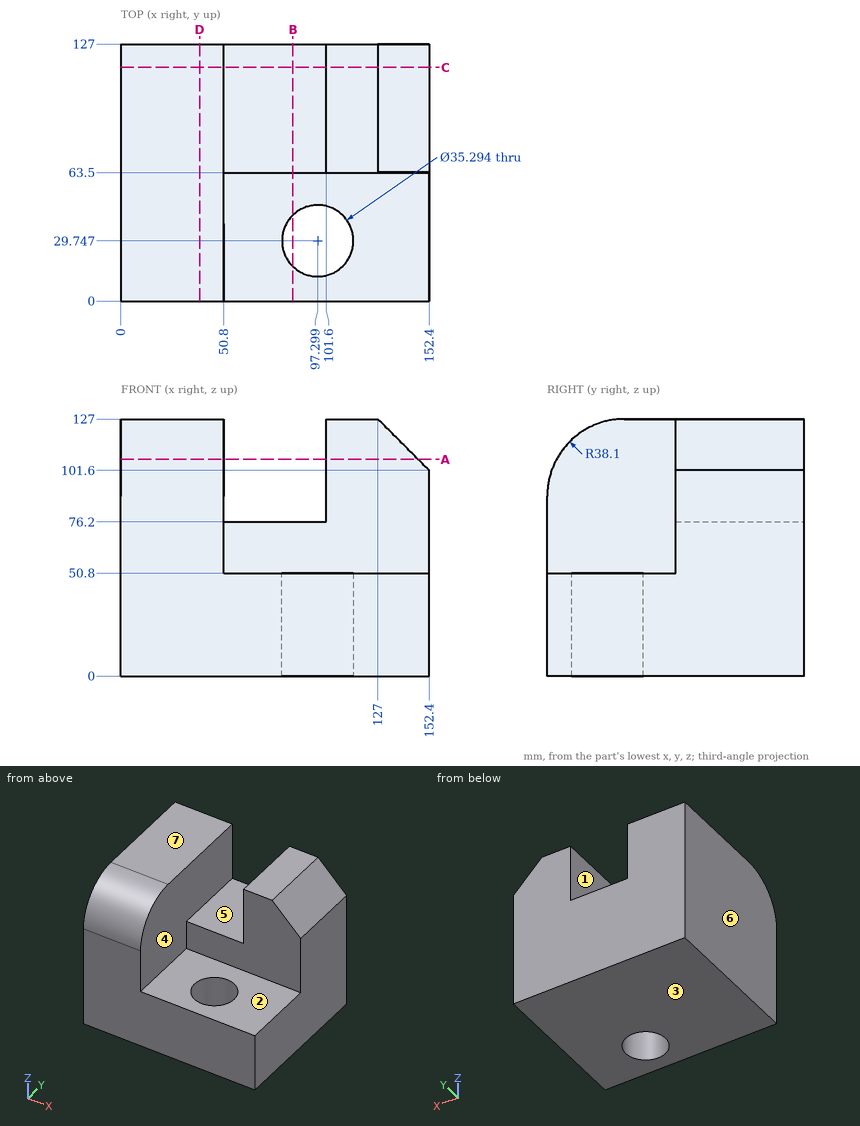
Check sheet for the drawn part. Datum: minimum x, y, z corner. Units: mm. A direction names the side the tool comes from. Coordinates: 2 decimals unless noted, no trailing zeros. Order: outer loops, then holes, each group sorted by start corner. A loop starts at its lowest first (then second) coordinate and runs counter-clockwise, first axis right, second up. Notation, with made-up numbers: M 51.5,-27 L 90.5,-27 A10 cw 90.5,-17 Z; hole C 21.25,89 d10. An arc over 180 degrees is marked long. One line per question, with ' | ' between items. Start each with the question number.
Item 1: Gauge pin test, flat end, axial feed: pin 1 (5 mm diameter, centred on x = 109, y = 47, fed in from +Z). Record the tip position at first contact, or that the pin passes through.
Item 2: Material ranges on L1, parallel to X at y = 100.5, z = 86; L2, parallel to Y at x = 116, z = 86.5; L3, parallel to X at y = 69, z = 113, recorded low to high. Write a range as [from, to].
Item 3: Draft check along X on the marked faces 5, 6 and 7. Enter one of: pulls with the +X half, pulls with the -X half, needs draft (parallel to the pull), parting line crosses it, or undercut.
Item 4: Cross-section at C-C on y = 115.5. Enter the section's corners in (x, z).
Item 5: Cross-section at A-A on z = 107. Enter the section's corners in (x, y), then the cut area to 3 significant figures.
Item 6: Cross-section at B-B on x = 85. Enter the section's corners in (y, z).
Item 7: Cross-section at D-D on x = 39. Enter the section's corners in (y, z), then the cut area to 3 significant figures.
Item 8: Set-up check for the marked faces 1, 2, 3 and 4: record each of +Z, -Z, +X, -X, +Y, -Y from which the full face is reachable in a straight line by a thin tool's end or side.
Findings:
1) pin 1: stops at z = 50.8
2) L1: x = [0, 50.8], [101.6, 152.4] | L2: y = [63.5, 127] | L3: x = [0, 50.8], [101.6, 141]
3) face 5: undercut | face 6: pulls with the -X half | face 7: needs draft
4) outline: M 0,0 L 152.4,0 L 152.4,101.6 L 127,127 L 101.6,127 L 101.6,76.2 L 50.8,76.2 L 50.8,127 L 0,127 Z
5) outline: M 0,4.57 L 50.8,4.57 L 50.8,127 L 0,127 Z; M 101.6,63.5 L 147,63.5 L 147,127 L 101.6,127 Z | area: 9,100 mm²
6) outline: M 0,0 L 17.09,0 L 17.09,50.8 L 0,50.8 Z; M 42.4,0 L 127,0 L 127,76.2 L 63.5,76.2 L 63.5,50.8 L 42.4,50.8 Z
7) outline: M 0,0 L 127,0 L 127,127 L 38.1,127 A38.1 ccw 0,88.9 Z | area: 15,800 mm²
8) face 1: +Z, +Y, -Y | face 2: +Z, +X, -Y | face 3: -Z, +X, -X, +Y, -Y | face 4: +Z, -Y
